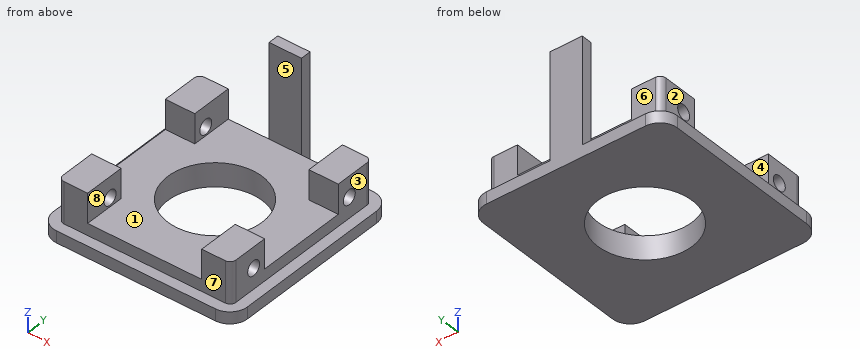
from build123d import *

# Parameters (mm, degrees)
F0_W      = 33
F0_H      = 33
F1_DEPTH  = 2
F2_W      = 29.4
F2_H      = 29.4
F3_DEPTH  = 2
F4_W      = 5
F4_H      = 7
F5_DEPTH  = 5
F6_R      = 8
F7_DEPTH  = 25
F8_R      = 1.25
F9_DEPTH  = 35
F10_R     = 1
F11_R     = 3
F12_W     = 5.5
F12_H     = 1.8
F13_DEPTH = 18


with BuildPart() as f1:
    # F0 (on Top) → F1 (new body)
    with BuildSketch(Plane.XY):
        with Locations((16.5, -16.5)):
            Rectangle(F0_W, F0_H)
    extrude(amount=F1_DEPTH)

    # F2 (on face) → F3 (join)
    with BuildSketch(Plane.XY.offset(2)):
        with Locations((16.5, -16.5)):
            Rectangle(F2_W, F2_H)
    extrude(amount=F3_DEPTH)

    # F4 (on face) → F5 (join)
    with BuildSketch(Plane.XY.offset(4)):
        with Locations((4.3, -5.3)):
            Rectangle(F4_W, F4_H)
        with Locations((4.3, -27.7)):
            Rectangle(F4_W, F4_H)
        with Locations((28.7, -5.3)):
            Rectangle(F4_W, F4_H)
        with Locations((28.7, -27.7)):
            Rectangle(F4_W, F4_H)
    extrude(amount=F5_DEPTH)

    # F6 (on face) → F7 (cut)
    with BuildSketch(Plane(origin=(0, 0, 0), x_dir=(1, 0, 0), z_dir=(0, 0, -1))):
        with Locations((16.5, 16.5)):
            Circle(F6_R)
    extrude(amount=-F7_DEPTH, mode=Mode.SUBTRACT)

    # F8 (on face) → F9 (cut)
    with BuildSketch(Plane.YZ.offset(31.2)):
        with Locations((-26.5, 5.5)):
            Circle(F8_R)
        with Locations((-6.5, 5.5)):
            Circle(F8_R)
    extrude(amount=-F9_DEPTH, mode=Mode.SUBTRACT)

    # F10
    f10_edges = [f1.edges().sort_by_distance(p)[0] for p in [
        (31.2, -1.8, 5.5),
        (1.8, -1.8, 5.5),
        (1.8, -31.2, 5.5),
        (31.2, -31.2, 5.5),
    ]]
    fillet(f10_edges, radius=F10_R)

    # F11
    f11_edges = [f1.edges().sort_by_distance(p)[0] for p in [
        (0, -33, 1),
        (33, -33, 1),
        (0, 0, 1),
        (33, 0, 1),
    ]]
    fillet(f11_edges, radius=F11_R)

    # F12 (on face) → F13 (join)
    with BuildSketch(Plane.XY.offset(2)):
        with Locations((16.5, -0.9)):
            Rectangle(F12_W, F12_H)
    extrude(amount=F13_DEPTH)


solid = f1.part
Design review of the part built by this model. Coordinates are the model's own, in mm. Face numbers are marked on the shaded views. A direction names the side the tool comes from. Give positions to 0.01 mm unless a question says otherwise; leave off trailing zeros. Write each loop counter-clockwise with the first axis right and the second up, starting at its lowest first coordinate (ties: lowest second). Pieces come first, ordered by that corner, then holes. Notation, with made-up numbers: M 11.25,-34 L 69.25,-34 A32 ccw 69.25,1 Z; hole C -29,30 d11. An arc over 180 degrees is marked long. Return JSON: item names as keys, results as strings. Group by question number.
Item 1: Take a section at B-B (x = 16.5). Give the boundary of the cut face in (y, z), plus the area to 3 significant figures.
Item 2: Wall thickness on line 1 along X through (y, z) = (-16.5, 1.25); line 2 along Z through (x, y) = (27.2, -26.5); line 3 along Y through (x, z) = (16.5, 1.5): over which ranges is each line inside the solid? List them lowest first.
Item 3: Take a section at A-A (y = -6.5). Give the boundary of the cut face in (x, z).
Item 4: Take a section at C-C (x = 5). Give the boundary of the cut face in (y, z), plus the area to 3 significant figures.
Item 5: Clearance check with flat-ended pins moving along their axes: pin 1 Ø12 at (y, z) = (-3.5, 17.5) entering from +X; pin 2 Ø1.5 at (x, y) = (5, -3.5) entering from +Z; pin 3 Ø10 at (y, z) = (-29, 10) entering from -X. State where each tip first meets the part, or that it passes through.
Item 6: The part is to be moulded in two halves that separate along X. For the marked faces 1, 2, 3 and 4, say which applies: pulls with the +X half, pulls with the -X half, needs draft (parallel to the pull), parting line crosses it, or undercut.
Item 7: Take a section at D-D (z = 5.5). Count the separate pieces of the cut face and the enclosed holes in it, plus the area to 3 significant figures.
Item 8: Tool access review of the marked faces 5, 6, 7 and 8: name each direction out of +Z, -Z, +X, -X, +Y, -Y from which nothing blocks a thin tool from reaching the whole face with its end or side.
Return value:
{
 "1": {"outline": "M -33,0 L -24.5,0 L -24.5,4 L -31.2,4 L -31.2,2 L -33,2 Z; M -8.5,0 L 0,0 L 0,20 L -1.8,20 L -1.8,4 L -8.5,4 Z", "area": "93.2 mm2"},
 "2": {"line 1": "x = 0 to 8.5, 24.5 to 33", "line 2": "z = 0 to 4.25, 6.75 to 9", "line 3": "y = -33 to -24.5, -8.5 to 0"},
 "3": {"outline": "M 0,0 L 33,0 L 33,2 L 31.2,2 L 31.2,4.25 L 26.2,4.25 L 26.2,4 L 6.8,4 L 6.8,4.25 L 1.8,4.25 L 1.8,2 L 0,2 Z; M 1.8,6.75 L 6.8,6.75 L 6.8,9 L 1.8,9 Z; M 26.2,6.75 L 31.2,6.75 L 31.2,9 L 26.2,9 Z"},
 "4": {"outline": "M -33,0 L 0,0 L 0,2 L -1.8,2 L -1.8,9 L -8.8,9 L -8.8,4 L -24.2,4 L -24.2,9 L -31.2,9 L -31.2,2 L -33,2 Z; hole C -26.5,5.5 d2.5; hole C -6.5,5.5 d2.5", "area": "185 mm2"},
 "5": {"pin 1": "stops at x = 19.25", "pin 2": "stops at z = 9", "pin 3": "stops at x = 1.8"},
 "6": {"face 1": "undercut", "face 2": "pulls with the -X half", "face 3": "pulls with the +X half", "face 4": "needs draft"},
 "7": {"separate pieces": "9", "enclosed holes": "0", "area": "99.0 mm2"},
 "8": {"face 5": "+Z, -Y", "face 6": "+Z, -X, +Y", "face 7": "+Z, +X, -X, -Y", "face 8": "+Z, +Y, -Y"}
}
